Design review of the part built by this model. Coordinates are the model's own, in mm. A direction names the side the tool comes from. Coordinates: 2 decimals unless noted, no trailing zeros. Loops run counter-clockwise (first coordinate to the right, second up) from the corner with the lowest first, then second, coordinate; pieces in that order, holes last. Notation, with made-up numbers: (58, 57) -> (117, 57) arc R3 ccw to (117, 62) -> close; hole circle Ø11 at (-27.75, -28.5). An arc over 180 degrees is marked (long way). Use a Markdown table: item, result. Add a question column.
Q1. For probe 1 along X at (y, z) = (-19.25, 3); probe 2 along Y at (x, z) = (-12.7, 2) (3 decimals); probe 3 along Y at (x, z) = (-12.7, 7.5) (3 decimals), list the stretches that pass through material, from the lowest coordinate up.
Q2. Take a section at D-D on x = -13.5. Write out the cut boundary in (y, z) (3 decimals).
Q3. Draft analysis for pull direction X (two halves, no side actions). For faces 1 (the face through (22.5, -19, 5)), 2 (the face through (0, -24.105, 5)), 3 (the face through (13.749, -21.066, 4.696)), 4 (the face through (-11.651, -21.066, 4.696)), state which applies: pulls with the +X half, pulls with the -X half, needs draft (parallel to the pull), parting line crosses it, or undercut.
Q4. Clearance check with a flat-ended pin moving along its axis: pin 1 Ø1.6 at (x, y) = (-10.5, -14.5) entering from -Z. State where the tip first meets the part, or that it passes through.
Q5. Take a section at B-B on x = 12.7. Write out the cut boundary in (y, z) (3 decimals).
Q6. For faces 5 (the face through (0, -15.555, 2)), 6 (the face through (-22.5, -19, 5)), list the 3-axis set-ups (+Z, -Z, +X, -X, +Y, -Y) from which the entire face can be reached by the end or side of a thin tool; tool diameter is ignored.
Q7. Take a section at C-C on z = 0.5. Write out the cut boundary in (x, y) (3 decimals), plus the area to 3 significant figures.
Q8. Take a section at A-A on y = -19.05. Write out the cut boundary in (x, z) (3 decimals), plus the area to 3 significant figures.
from build123d import *

# Parameters (mm, degrees)
BOSS_EXTRUDE1_DEPTH  = 22.5
MOUNTHOLES_SKETCH_R  = 2.2729
MOUNTHOLES_CUT_DEPTH = 35.322392836


with BuildPart() as part:
    # yExtentCalculator_sketch → Boss-Extrude1 (new, symmetric)
    with BuildSketch(Plane(origin=(0, 0, 0), x_dir=(0, 0, -1), z_dir=(1, 0, 0))):
        Polygon((-9.525, -14.105), (-9.525, -24.105), (0, -24.105), (0, -15.555), (-4.32, -15.555), (-4.32, -14.105), align=None)
    extrude(amount=BOSS_EXTRUDE1_DEPTH, both=True)

    # mountHoles_sketch → mountHoles_cut (cut, through all)
    with BuildSketch(Plane.XY):
        with Locations((12.7, -19.05)):
            Circle(MOUNTHOLES_SKETCH_R)
        with Locations((-12.7, -19.05)):
            Circle(MOUNTHOLES_SKETCH_R)
    extrude(amount=MOUNTHOLES_CUT_DEPTH, mode=Mode.SUBTRACT)


solid = part.part
Answer list:
| question | item | result |
|---|---|---|
| 1 | probe 1 | -22.5 to -14.96, -10.44 to 10.44, 14.96 to 22.5 |
| 1 | probe 2 | -24.105 to -21.323, -16.777 to -15.555 |
| 1 | probe 3 | -24.105 to -21.323, -16.777 to -14.105 |
| 2 | outline | (-24.105, 0) -> (-21.177, 0) -> (-21.177, 9.525) -> (-24.105, 9.525) -> close; (-16.923, 0) -> (-15.555, 0) -> (-15.555, 4.32) -> (-14.105, 4.32) -> (-14.105, 9.525) -> (-16.923, 9.525) -> close |
| 3 | face 1 | pulls with the +X half |
| 3 | face 2 | needs draft |
| 3 | face 3 | undercut |
| 3 | face 4 | undercut |
| 4 | pin 1 | z = 4.32 |
| 5 | outline | (-24.105, 0) -> (-21.323, 0) -> (-21.323, 9.525) -> (-24.105, 9.525) -> close; (-16.777, 0) -> (-15.555, 0) -> (-15.555, 4.32) -> (-14.105, 4.32) -> (-14.105, 9.525) -> (-16.777, 9.525) -> close |
| 6 | face 5 | -Z, +X, -X, +Y |
| 6 | face 6 | +Z, -Z, -X, +Y, -Y |
| 7 | outline | (-22.5, -24.105) -> (22.5, -24.105) -> (22.5, -15.555) -> (-22.5, -15.555) -> close; hole circle Ø4.546 at (-12.7, -19.05); hole circle Ø4.546 at (12.7, -19.05) |
| 7 | area | 352 mm² |
| 8 | outline | (-22.5, 0) -> (-14.973, 0) -> (-14.973, 9.525) -> (-22.5, 9.525) -> close; (-10.427, 0) -> (10.427, 0) -> (10.427, 9.525) -> (-10.427, 9.525) -> close; (14.973, 0) -> (22.5, 0) -> (22.5, 9.525) -> (14.973, 9.525) -> close |
| 8 | area | 342 mm² |
